```python
from build123d import *

# Parameters (mm, degrees)
TRAY_SKETCH_R   = 97
TRAY_SKETCH_R_2 = 1.7
TRAY_SKETCH_R_3 = 1.35
TRAY_SKETCH_W   = 15
TRAY_SKETCH_H   = 3
TRAY_DEPTH      = 3.18


with BuildPart() as part:
    # Tray Sketch → Tray (new body)
    with BuildSketch(Plane(origin=(0, 0, 0), x_dir=(0, 0, -1), z_dir=(1, 0, 0))):
        with Locations(Location((0, 0, 0), (0, 0, 180))):
            Circle(TRAY_SKETCH_R)
        with Locations(Location((0, 92, 0), (0, 0, 180))):
            Circle(TRAY_SKETCH_R_2, mode=Mode.SUBTRACT)
        with Locations(Location((-92, 0, 0), (0, 0, 180))):
            Circle(TRAY_SKETCH_R_2, mode=Mode.SUBTRACT)
        with Locations(Location((0, -92, 0), (0, 0, 180))):
            Circle(TRAY_SKETCH_R_2, mode=Mode.SUBTRACT)
        with Locations(Location((92, 0, 0), (0, 0, 180))):
            Circle(TRAY_SKETCH_R_2, mode=Mode.SUBTRACT)
        with Locations(Location((32, -50, 0), (0, 0, 180))):
            Circle(TRAY_SKETCH_R_2, mode=Mode.SUBTRACT)
        with Locations(Location((-32, -50, 0), (0, 0, 180))):
            Circle(TRAY_SKETCH_R_2, mode=Mode.SUBTRACT)
        with Locations(Location((32, 50, 0), (0, 0, 180))):
            Circle(TRAY_SKETCH_R_2, mode=Mode.SUBTRACT)
        with Locations(Location((-32, 50, 0), (0, 0, 180))):
            Circle(TRAY_SKETCH_R_2, mode=Mode.SUBTRACT)
        with Locations(Location((62, -24, 0), (0, 0, 180))):
            Circle(TRAY_SKETCH_R_3, mode=Mode.SUBTRACT)
        with Locations(Location((62, 24, 0), (0, 0, 180))):
            Circle(TRAY_SKETCH_R_3, mode=Mode.SUBTRACT)
        with Locations(Location((81, 0, 0), (0, 0, 180))):
            Circle(TRAY_SKETCH_R_3, mode=Mode.SUBTRACT)
        Polygon((32.526911935, -60.811183182), (60.811183182, -32.526911935), (73.539105243, -45.254833996), (45.254833996, -73.539105243), align=None, mode=Mode.SUBTRACT)
        with Locations((-30, 6)):
            Rectangle(TRAY_SKETCH_W, TRAY_SKETCH_H, mode=Mode.SUBTRACT)
        with Locations((-30, 44)):
            Rectangle(TRAY_SKETCH_W, TRAY_SKETCH_H, mode=Mode.SUBTRACT)
        with Locations((30, 6)):
            Rectangle(TRAY_SKETCH_W, TRAY_SKETCH_H, mode=Mode.SUBTRACT)
        with Locations((30, 44)):
            Rectangle(TRAY_SKETCH_W, TRAY_SKETCH_H, mode=Mode.SUBTRACT)
        with Locations((-20, -43)):
            Rectangle(TRAY_SKETCH_W, TRAY_SKETCH_H, mode=Mode.SUBTRACT)
        with Locations((-20, -6)):
            Rectangle(TRAY_SKETCH_W, TRAY_SKETCH_H, mode=Mode.SUBTRACT)
        with Locations((20, -43)):
            Rectangle(TRAY_SKETCH_W, TRAY_SKETCH_H, mode=Mode.SUBTRACT)
        with Locations((20, -6)):
            Rectangle(TRAY_SKETCH_W, TRAY_SKETCH_H, mode=Mode.SUBTRACT)
        with Locations((-62, -43.5)):
            Rectangle(TRAY_SKETCH_W, TRAY_SKETCH_H, mode=Mode.SUBTRACT)
        with Locations((-62, 3.5)):
            Rectangle(TRAY_SKETCH_W, TRAY_SKETCH_H, mode=Mode.SUBTRACT)
    extrude(amount=TRAY_DEPTH)


solid = part.part
```
Verification items for the finished model (mm, model axes). A direction names the side the tool comes from. Coordinates: 2 decimals unless noted, no trailing zeros. Loops run counter-clockwise (first coordinate to the right, second up) from the corner with the lowest first, then second, coordinate; pieces in that order, holes last. Notation, with made-up numbers: (13, -0.5) -> (21, -0.5) arc R29 cw to (21, 25.5) -> close; hole circle Ø3 at (-33.5, -20). An arc over 180 degrees is marked (long way). Answer in a Markdown table with one row per item. Add a question column.
1. Section check C-C, the plane x = 0.7. Give the number of separate pieces and of enclosed holes in the cut face, then the cut area to 3 significant figures.
2. Section check B-B, the plane y = -37.5. Enter the section's corners in (x, z).
3. Draft check along Y on faces 1 (the face through (1.568, -67.264, -38.98)), 2 (the face through (1.568, 86.056, 44.76)), 3 (the face through (0, -1, -1)). Enter one of: +Y half, -Y half, draft (parallel to the pull), parting line (faces both ways), or undercut.
4. Material ranges on probe 1 along Z at (x, y) = (1.6, -50); probe 2 along Y at (x, z) = (2.4, -32); probe 3 along Y at (x, z) = (3.05, -80), recorded low to high. Write a range as [from, to].
5. Depth check by flat-ended pin: P1, Ø1, axis at x = 1, z = 29.5, coming from the +Y side; P2, Ø1, axis at x = 1, y = -42, coming from the +Z side; P3, Ø1.6, axis at x = 2, z = 33.5, coming from the -Y side; P4, Ø3, axis at y = -62.5, z = 71, coming from the -X side. Enter the tip coordinate at first touch or a pass-through.
6. Section check D-D, the plane z = 16. Enter the section's corners in (x, y).
7. Access from +Z, -Z, +X, -X, +Y, -Y to the whole of each face (thin tool, end or side, straight path). Record for faces 4 (the face through (1.568, -38.802, -67.086)), 5 (the face through (3.18, -1, -1)).
8. Section check A-A, the plane z = 60.5. Enter the section's corners in (x, y).
Derived:
| question | item | result |
|---|---|---|
| 1 | separate pieces | 1 |
| 1 | enclosed holes | 22 |
| 1 | area | 28,300 mm² |
| 2 | outline | (0, -89.46) -> (3.18, -89.46) -> (3.18, -65.78) -> (0, -65.78) -> close; (0, -55.84) -> (3.18, -55.84) -> (3.18, 89.46) -> (0, 89.46) -> close |
| 3 | face 1 | undercut |
| 3 | face 2 | parting line |
| 3 | face 3 | draft |
| 4 | probe 1 | z = [-83.12, -68.79], [-43.34, -33.7], [-30.3, 30.3], [33.7, 83.12] |
| 4 | probe 2 | y = [-91.57, -51.7], [-48.3, 4.5], [7.5, 42.5], [45.5, 48.3], [51.7, 91.57] |
| 4 | probe 3 | y = [-54.85, -0.91], [0.91, 54.85] |
| 5 | P1 | stops at y = 92.56 |
| 5 | P2 | stops at z = 87.67 |
| 5 | P3 | stops at y = -91.32 |
| 5 | P4 | stops at x = 0 |
| 6 | outline | (0, -95.67) -> (3.18, -95.67) -> (3.18, -44.5) -> (0, -44.5) -> close; (0, -41.5) -> (3.18, -41.5) -> (3.18, -7.5) -> (0, -7.5) -> close; (0, -4.5) -> (3.18, -4.5) -> (3.18, 95.67) -> (0, 95.67) -> close |
| 7 | face 4 | +X, -X |
| 7 | face 5 | +Z, -Z, +X, +Y, -Y |
| 8 | outline | (0, -75.82) -> (3.18, -75.82) -> (3.18, -45) -> (0, -45) -> close; (0, -42) -> (3.18, -42) -> (3.18, 2) -> (0, 2) -> close; (0, 5) -> (3.18, 5) -> (3.18, 75.82) -> (0, 75.82) -> close |
